Could you check a few things on this model? Use its own coordinates, in mm. A direction names the side the tool comes from. Round coordinates to 2 decimals unless told otherwise and drop trailing zeros. Loops run counter-clockwise (first coordinate to the right, second up) from the corner with the lowest first, then second, coordinate; pieces in that order, holes last. Notation, with made-up numbers: (8.5, 60.5) -> (37.5, 60.5) arc R21 ccw to (37.5, 74.5) -> close; hole circle Ø11 at (-4.75, 46). An arc over 180 degrees is marked (long way). One line per item, written item: value.
Autodesk Inventor part; units mm, degrees
ref_plane "Plan de construction2" through (14, 0, 0) normal (1, 0, 0) x (0, 1, 0)
ref_plane "Plan de construction3" through (11, 0, 23) normal (1, 0, 0) x (0, 1, 0)
ref_plane "XZ Plane" through (0, 0, 0) normal (0, 1, 0) x (-1, 0, 0)
sketch "Esquisse1" plane through (0, 0, 0) normal (1, 0, 0) x (0, 1, 0)
  line L0 (0, 0) -> (0, 17.1522)
  line L1 (8, 50) -> (8, 36)
  line L2 (8, 36) -> (6, 36)
  line L3 (6, 36) -> (6, 30)
  line L4 (6, 30) -> (8, 24.505)
  line L5 (8, 24.505) -> (8, 1)
  line L6 (8, 1) -> (9, 0)
  line L7 (9, 0) -> (10, 0)
  line L8 (8, 50) -> (9, 50)
  line L9 (9, 50) -> (11, 45)
  line L10 (11, 45) -> (11, 1)
  line L11 (11, 1) -> (10, 0)
  dimension "d0" = 160
  dimension "d1" = 6
  dimension "d2" = 14
  dimension "d4" = 16
  dimension "d6" = 16
  dimension "d8" = 1
  dimension "d9" = 1
  dimension "d10" = 30
  dimension "d11" = 1
  dimension "d12" = 2
  dimension "d13" = 22
  dimension "d14" = 3
  dimension "d15" = 5
  dimension "d19" = 1
  dimension "d20" = 1
revolve "Révolution1" add sketch "Esquisse1" angle 360 about axis through (0, 0, 0) along (0, 0, 1)
thread "Filetage1"
ref_plane "Plan de construction2" through (14, 0, 0) normal (1, 0, 0) x (0, 1, 0)
sketch "Esquisse2" plane through (14, 0, 0) normal (1, 0, 0) x (0, 1, 0)
  circle A0 centre (0, 10) radius 2.5
  point P0 (0, 0)
  dimension "d22" = 5
  dimension "d23" = 10
extrude "Extrusion1" add sketch "Esquisse2" against normal up to surface
chamfer "Chanfrein1" distance 0.5 angle 45 2 edges at (10.7122, -2.5, 10.0138) (14, -2.5, 10)
pattern_circular "Réseau circulaire1" count 2 over 360 about axis through (0, 0, -10) along (0, 0, 1) of "Extrusion1", "Chanfrein1"
ref_plane "Plan de construction3" through (11, 0, 23) normal (1, 0, 0) x (0, 1, 0)
sketch "Esquisse4" plane through (11, 0, 23) normal (1, 0, 0) x (0, 1, 0)
  line L0 (0, 31) -> (0, 1) construction
  line L1 (1.5, 31) -> (1.5, 1)
  line L2 (-1.5, 1) -> (-1.5, 31)
  arc A0 (1.5, 31) -> (-1.5, 31) centre (0, 31) ccw
  arc A1 (-1.5, 1) -> (1.5, 1) centre (0, 1) ccw
  line L3 (-11, 22) -> (11, 22)
  point P0 (0, -23)
  point P1 (0, 16)
  dimension "d39" = 1.5
  dimension "d40" = 30
  dimension "d47" = 24
extrude "Extrusion2" cut sketch "Esquisse4" against normal blind 1
chamfer "Chanfrein3" distance 0.5 angle 45 4 edges at (10.8972, 1.5, 34.5) (10.9487, -1.0614, 22.9401) (10.9417, 1.131, 23.0147) (10.8972, -1.5, 34.5)
properties part number "support_douille" material "Aluminium 6061"
Item 1: Will these pins go through, and if not, where does the flat tip stop? pin 1 Ø9.5 at (x, y) = (0, 0) entering from +Z; pin 2 Ø8 at (x, y) = (-0.5, 3.5) entering from +Z; pin 3 Ø8 at (x, z) = (8, 44) entering from +Y; pin 4 Ø1.5 at (x, z) = (-6.5, 42) entering from +Y.
Output:
pin 1: passes through
pin 2: stops at z = 36
pin 3: stops at y = 10.25
pin 4: stops at y = 9.38
Item 2: If we section it at A-A on x = 0: List the corners of the cut face in (y, z) for me (3 decimals), plus the area to 3 significant figures.
Output:
outline: (-11, 1) -> (-10, 0) -> (-9, 0) -> (-8, 1) -> (-8, 24.505) -> (-6, 30) -> (-6, 36) -> (-8, 36) -> (-8, 50) -> (-9, 50) -> (-11, 45) -> close; (6, 30) -> (8, 24.505) -> (8, 1) -> (9, 0) -> (10, 0) -> (11, 1) -> (11, 45) -> (9, 50) -> (8, 50) -> (8, 36) -> (6, 36) -> close
area: 323 mm²
Item 3: If we section it at D-D on z = 33.5: List the corners of the cut face in (x, y) for me, plus the area to 3 significant figures.
Output:
outline: (10, -1.5) -> (10, 1.5) -> (10.4, 1.5) -> (10.82, 1.99) arc R11 ccw (long way) to (10.82, -1.99) -> (10.4, -1.5) -> close; hole circle Ø12 at (0, 0)
area: 264 mm²
Item 4: If we section it at C-C on x = 12: List the corners of the cut face in (y, z) for me.
Output:
outline: circle Ø5 at (0, 10)
Item 5: For faces 4 (the face through (-6, -2, 36)), 5 (the face through (12.4, -2.5, 10.1)), 6 (the face through (10, 0, 35)), 7 (the face through (-12.4, 2.5, 10.1)), 8 (the face through (0, -6, 33)), which set-ups out of +Z, -Z, +X, -X, +Y, -Y let a thin tool reach every point of the face, with its end or its side?
Output:
face 4: +Z
face 5: +X
face 6: +Z, +X
face 7: -X
face 8: +Z, -Z
Item 6: If we mould it in two halves opening along X, with no side actions, what happens to faces 1 (the face through (-8.9, -2, 49.7)), 2 (the face through (14, 0, 10)), 3 (the face through (-7.81, -1.73, 12.59))? For each: released by +X, released by -X, zero draft, split by the parting line, or undercut.
Output:
face 1: split by the parting line
face 2: released by +X
face 3: undercut
Item 7: If we section it at B-B on z = 39.5: List the corners of the cut face in (x, y) for me, plus the area to 3 significant figures.
Output:
outline: (10, -1.5) -> (10, 1.5) -> (10.4, 1.5) -> (10.82, 1.99) arc R11 ccw (long way) to (10.82, -1.99) -> (10.4, -1.5) -> close; hole circle Ø16 at (0, 0)
area: 176 mm²
Item 8: I need wall thicknesses on line 1 (Y direction, x = 0, z = 19); line 2 (X direction, y = 0, z = 33.65); line 3 (Y direction, x = 0, z = 34.5). Which ranges of each line are inside material? Lowest first, please. Write a range as from..to.
Output:
line 1: y = -11..-8, 8..11
line 2: x = -11..-6, 6..10
line 3: y = -11..-6, 6..11
